from build123d import *

# Parameters (mm, degrees)
SKETCH1_R           = 12.5
SKETCH1_R_2         = 7.5
BOSS_EXTRUDE1_DEPTH = 3
SKETCH2_R           = 14
SKETCH2_R_2         = 7.5
BOSS_EXTRUDE2_DEPTH = 3
BOSS_EXTRUDE2_TAPER = 30
SKETCH3_R           = 14
SKETCH3_R_2         = 7.5
BOSS_EXTRUDE3_DEPTH = 3
BOSS_EXTRUDE3_TAPER = 30


with BuildPart() as part:
    # Sketch1 → Boss-Extrude1 (new body)
    with BuildSketch(Plane.XY):
        Circle(SKETCH1_R)
        Circle(SKETCH1_R_2, mode=Mode.SUBTRACT)
    extrude(amount=BOSS_EXTRUDE1_DEPTH)

    # Sketch2 → Boss-Extrude2 (add)
    with BuildSketch(Plane.XY.offset(3)):
        Circle(SKETCH2_R)
        Circle(SKETCH2_R_2, mode=Mode.SUBTRACT)
    extrude(amount=BOSS_EXTRUDE2_DEPTH, taper=BOSS_EXTRUDE2_TAPER)

    # Sketch3 → Boss-Extrude3 (add)
    with BuildSketch(Plane(origin=(0, 0, 0), x_dir=(-1, 0, 0), z_dir=(0, 0, -1))):
        Circle(SKETCH3_R)
        Circle(SKETCH3_R_2, mode=Mode.SUBTRACT)
    extrude(amount=BOSS_EXTRUDE3_DEPTH, taper=BOSS_EXTRUDE3_TAPER)


solid = part.part
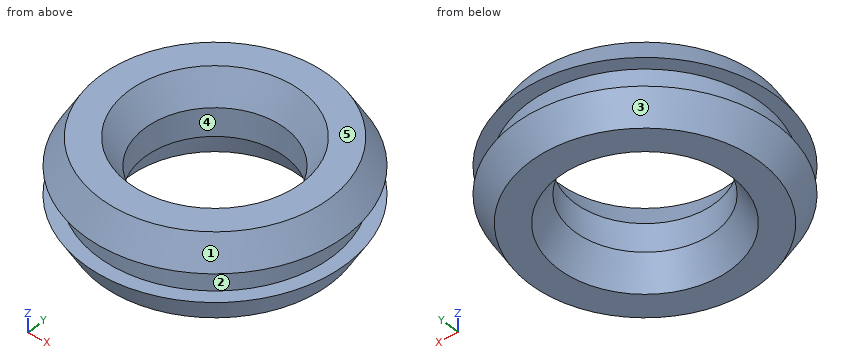
Can you work these out from the model? Positions are in its coordinate system, mm. Face numbers are marked on the shaded views. A direction names the side the tool comes from. Give positions to 0.01 mm unless a question says otherwise; leave off trailing zeros. Order: outer loops, then holes, each group sorted by start corner. A loop starts at its lowest first (then second) coordinate and runs counter-clockwise, first axis right, second up. Notation, with made-up numbers: M 85.25,86.25 L 124.25,86.25 A21 cw 124.25,111.25 Z; hole C 19.25,-35 d6. An arc over 180 degrees is marked long. Use a Markdown table: item, result. Add a question column.
Item 1: Suppose I cut it at C-C (z = -1.75). List the corners of the cut face in (x, y) for me.
Item 2: If I drill on L1, parallel to Y at x = 0, z = 0.7; L2, parallel to Z at x = 10.75, y = 8.5; L3, parallel to Z at x = -12.75, y = -0.25, over which ranges is the centre line in solid material (lowest first)? Write a range as [from, to].
Item 3: For the marked faces 1 and 2, which set-ups out of +Z, -Z, +X, -X, +Y, -Y let a thin tool reach every point of the face, with its end or its side?
Item 4: Suppose I cut it at B-B (z = 0.5). List the corners of the cut face in (x, y) for me, then the cut area to 3 significant figures.
Item 5: Will these pins go through, and if not, where does the flat tip stop? pin 1 (2 mm diameter, centred on y = -5.5, z = 1.5, fed in from +X); pin 2 (1 mm diameter, centred on y = -4.5, z = 4, fed in from +X); pin 3 (1 mm diameter, centred on x = -10.5, z = -1, fed in from +Y).
Item 6: Suppose I cut it at A-A (x = 0). List the corners of the cut face in (y, z) for me.
Item 7: We'd pull the mould along X, two halves only. Please class the marked faces 3, 4 and 5: +X half, -X half, draft (parallel to the pull), parting line (faces both ways), or undercut.
Answer sheet:
| question | item | result |
|---|---|---|
| 1 | outline | C 0,0 d25.98; hole C 0,0 d17.02 |
| 2 | L1 | y = [-12.5, -7.5], [7.5, 12.5] |
| 2 | L2 | z = [-0.51, 0], [3, 3.51] |
| 2 | L3 | z = [-2.16, 0], [3, 5.16] |
| 3 | face 1 | +Z |
| 3 | face 2 | none |
| 4 | outline | C 0,0 d25; hole C 0,0 d15 |
| 4 | area | 314 mm² |
| 5 | pin 1 | stops at x = 11.66 |
| 5 | pin 2 | stops at x = 13 |
| 5 | pin 3 | stops at y = 9.1 |
| 6 | outline | M -14,0 L -12.27,-3 L -9.23,-3 L -7.5,0 L -7.5,3 L -9.23,6 L -12.27,6 L -14,3 L -12.5,3 L -12.5,0 Z; M 7.5,0 L 9.23,-3 L 12.27,-3 L 14,0 L 12.5,0 L 12.5,3 L 14,3 L 12.27,6 L 9.23,6 L 7.5,3 Z |
| 7 | face 3 | parting line |
| 7 | face 4 | undercut |
| 7 | face 5 | draft |
